from build123d import *

# Parameters (mm, degrees)
SKETCH1_W           = 147
SKETCH1_H           = 95.25
BOSS_EXTRUDE1_DEPTH = 26
SKETCH2_R           = 1.5
CUT_EXTRUDE3_DEPTH  = 26


with BuildPart() as part:
    # Sketch1 → Boss-Extrude1 (new body)
    with BuildSketch(Plane(origin=(0, 0, 0), x_dir=(1, 0, 0), z_dir=(0, 1, 0))):
        with Locations((8.120065789, 8.250822368)):
            Rectangle(SKETCH1_W, SKETCH1_H)
    extrude(amount=BOSS_EXTRUDE1_DEPTH)

    # Sketch2 → Cut-Extrude3 (cut)
    with BuildSketch(Plane.XY.offset(39.374177632)):
        with Locations((-48.479934211, 6.35)):
            Circle(SKETCH2_R)
        with Locations((11.510065789, 6.35)):
            Circle(SKETCH2_R)
        with Locations((53.120065789, 6.35)):
            Circle(SKETCH2_R)
    extrude(amount=-CUT_EXTRUDE3_DEPTH, mode=Mode.SUBTRACT)


solid = part.part
Work out the finished part from the listing and answer in its coordinate system (mm). A direction names the side the tool comes from. Coordinates: 2 decimals unless noted, no trailing zeros. Write each loop counter-clockwise with the first axis right and the second up, starting at its lowest first coordinate (ties: lowest second). Pieces come first, ordered by that corner, then holes. Notation, with made-up numbers: (88.5, 16) - (113.5, 16) arc R27 ccw to (113.5, 54) - close; hole circle Ø4 at (36, 6.5). An arc over 180 degrees is marked (long way). One line per question, with ' | ' between items.
1) For faces 4 (the face through (51.93, 5.44, 26.56)), 5 (the face through (7, 26, -9)), determine the directions among +Z, -Z, +X, -X, +Y, -Y from which every point of the face is accessible in a straight line to the end or side of a thin tool.
Checks:
face 4: +Z | face 5: +Z, -Z, +X, -X, +Y
2) Consider probe 1 along Z at (x, y) = (-49, 7.5). Determine where the line is inside the solid, lowest interval first. Write a range as [from, to].
Checks:
probe 1: [-55.88, 13.37]
3) The mould has two halves that part along X. Classify faces 1 (the face through (11, 6, 13.374)), 2 (the face through (7, 13, -55.876)), 3 (the face through (-65.38, 13, -8)): +X half, -X half, draft (parallel to the pull), parting line (faces both ways), or undercut.
Checks:
face 1: undercut | face 2: draft | face 3: -X half
4) Find section A-A, the plane y = 6.35. Determine the outline of the cut face in (x, z).
Checks:
outline: (-65.38, -55.88) - (81.62, -55.88) - (81.62, 39.37) - (54.62, 39.37) - (54.62, 13.37) - (51.62, 13.37) - (51.62, 39.37) - (13.01, 39.37) - (13.01, 13.37) - (10.01, 13.37) - (10.01, 39.37) - (-46.98, 39.37) - (-46.98, 13.37) - (-49.98, 13.37) - (-49.98, 39.37) - (-65.38, 39.37) - close
